```python
from build123d import *

# Parameters (mm, degrees)
SKETCH1_R           = 9
BOSS_EXTRUDE1_DEPTH = 2
SKETCH1_4_W         = 2
SKETCH1_4_H         = 20
BOSS_EXTRUDE2_DEPTH = 8
SKETCH1_5_R         = 0.5
CUT_EXTRUDE1_DEPTH  = 1
CUT_EXTRUDE2_DEPTH  = 9
SKETCH4_R           = 0.5
SKETCH4_R_2         = 1.5
CUT_EXTRUDE5_DEPTH  = 1
SKETCH6_R           = 2.5
CUT_EXTRUDE6_DEPTH  = 10
CUT_EXTRUDE8_DEPTH  = 10


with BuildPart() as part:
    # Sketch1 → Boss-Extrude1 (new body)
    with BuildSketch(Plane(origin=(0, 0, 0), x_dir=(1, 0, 0), z_dir=(0, 1, 0))):
        with Locations(Location((0, 0, 0), (0, 0, 270))):
            Circle(SKETCH1_R)
    extrude(amount=BOSS_EXTRUDE1_DEPTH)

    # Sketch1_4 → Boss-Extrude2 (add)
    with BuildSketch(Plane(origin=(0, 0, 0), x_dir=(1, 0, 0), z_dir=(0, 1, 0))):
        with BuildLine():
            ThreePointArc((9, 0), (6.363961031, -6.363961031), (0, -9))
            Line((0, -9), (14.5, -9))
            Line((14.5, -9), (16.5, -9))
            Line((16.5, -9), (7.566878981, 4.872611465))
            ThreePointArc((7.566878981, 4.872611465), (8.634289514, 2.539496916), (9, 0))
        make_face()
        with Locations((15.5, -19)):
            Rectangle(SKETCH1_4_W, SKETCH1_4_H)
    extrude(amount=BOSS_EXTRUDE2_DEPTH)

    # Sketch1_5 → Cut-Extrude1 (cut)
    with BuildSketch(Plane(origin=(0, 0, 0), x_dir=(1, 0, 0), z_dir=(0, 1, 0))):
        with BuildLine():
            ThreePointArc((2, 1.5), (1.767766953, 1.767766953), (1.5, 2))
            Line((1.5, 2), (1.5, 6.5))
            ThreePointArc((1.5, 6.5), (0, 8), (-1.5, 6.5))
            Line((-1.5, 6.5), (-1.5, 2))
            ThreePointArc((-1.5, 2), (-1.767766953, 1.767766953), (-2, 1.5))
            Line((-2, 1.5), (-6.5, 1.5))
            ThreePointArc((-6.5, 1.5), (-8, 0), (-6.5, -1.5))
            Line((-6.5, -1.5), (-2, -1.5))
            ThreePointArc((-2, -1.5), (-1.767766953, -1.767766953), (-1.5, -2))
            Line((-1.5, -2), (-1.5, -6.5))
            ThreePointArc((-1.5, -6.5), (0, -8), (1.5, -6.5))
            Line((1.5, -6.5), (1.5, -2))
            ThreePointArc((1.5, -2), (1.767766953, -1.767766953), (2, -1.5))
            Line((2, -1.5), (6.5, -1.5))
            ThreePointArc((6.5, -1.5), (8, 0), (6.5, 1.5))
            Line((6.5, 1.5), (2, 1.5))
        make_face()
        with Locations(Location((0, -6.5, 0), (0, 0, 270))):
            Circle(SKETCH1_5_R, mode=Mode.SUBTRACT)
        with Locations(Location((6.5, 0, 0), (0, 0, 270))):
            Circle(SKETCH1_5_R, mode=Mode.SUBTRACT)
        with Locations(Location((0, 6.5, 0), (0, 0, 270))):
            Circle(SKETCH1_5_R, mode=Mode.SUBTRACT)
        with Locations(Location((-6.5, 0, 0), (0, 0, 270))):
            Circle(SKETCH1_5_R, mode=Mode.SUBTRACT)
    extrude(amount=CUT_EXTRUDE1_DEPTH, mode=Mode.SUBTRACT)

    # Sketch2 → Cut-Extrude2 (cut)
    with BuildSketch(Plane.XY.offset(9)):
        Polygon((0, 2), (14.5, 8), (0, 8), align=None)
    extrude(amount=-CUT_EXTRUDE2_DEPTH, mode=Mode.SUBTRACT)

    # Sketch4 → Cut-Extrude5 (cut)
    # profile 1 of 3: a face of its own
    with BuildSketch(Plane(origin=(16.5, 0, 0), x_dir=(0, 0, -1), z_dir=(1, 0, 0))):
        with BuildLine():
            Line((-28.5684803, 6.462476548), (-29, 6.5))
            Line((-29, 6.5), (-29, 1.5))
            Line((-29, 1.5), (-28.5684803, 1.537523452))
            ThreePointArc((-28.5684803, 1.537523452), (-27.085737838, 2.392019784), (-26.5, 4))
            ThreePointArc((-26.5, 4), (-27.085737838, 5.607980216), (-28.5684803, 6.462476548))
        make_face()
    # profile 2 of 3: a face of its own
    with BuildSketch(Plane(origin=(16.5, 0, 0), x_dir=(0, 0, -1), z_dir=(1, 0, 0))):
        with BuildLine():
            Line((-17.5, 5.5), (-28.5684803, 6.462476548))
            ThreePointArc((-28.5684803, 6.462476548), (-27.085737838, 5.607980216), (-26.5, 4))
            ThreePointArc((-26.5, 4), (-27.085737838, 2.392019784), (-28.5684803, 1.537523452))
            Line((-28.5684803, 1.537523452), (-17.5, 2.5))
            ThreePointArc((-17.5, 2.5), (-19, 4), (-17.5, 5.5))
        make_face()
        with Locations((-22.5, 4)):
            Circle(SKETCH4_R, mode=Mode.SUBTRACT)
        with Locations((-20, 4)):
            Circle(SKETCH4_R, mode=Mode.SUBTRACT)
    # profile 3 of 3: a face of its own
    with BuildSketch(Plane(origin=(16.5, 0, 0), x_dir=(0, 0, -1), z_dir=(1, 0, 0))):
        with Locations((-17.5, 4)):
            Circle(SKETCH4_R_2)
        with Locations((-17.5, 4)):
            Circle(SKETCH4_R, mode=Mode.SUBTRACT)
    extrude(amount=-CUT_EXTRUDE5_DEPTH, mode=Mode.SUBTRACT)

    # Sketch6 → Cut-Extrude6 (cut)
    with BuildSketch(Plane(origin=(15.5, 0, 0), x_dir=(0, 0, -1), z_dir=(1, 0, 0))):
        with Locations((-29, 4)):
            Circle(SKETCH6_R)
    extrude(amount=-CUT_EXTRUDE6_DEPTH, mode=Mode.SUBTRACT)

    # Sketch8 → Cut-Extrude8 (cut)
    with BuildSketch(Plane(origin=(16.5, 0, 0), x_dir=(0, 0, -1), z_dir=(1, 0, 0))):
        Polygon((-9, 8), (4.872611465, 2), (4.872611465, 8), align=None)
    extrude(amount=-CUT_EXTRUDE8_DEPTH, mode=Mode.SUBTRACT)


solid = part.part
```
CAD build for the part. Positions are in the model's coordinates, mm. A direction names the side the tool comes from. Round coordinates to 2 decimals unless told otherwise and drop trailing zeros. Write each loop counter-clockwise with the first axis right and the second up, starting at its lowest first coordinate (ties: lowest second). Pieces come first, ordered by that corner, then holes. Notation, with made-up numbers: (-36, -5.5) - (-31, -5.5) arc R13 cw to (-31, 6.5) - close; hole circle Ø10 at (-27, 87.25). An arc over 180 degrees is marked (long way). Write item = value, one per line. Start each with the question number.
Q1. Band-saw the part on C-C (x = -4.25). Give the cut face in (y, z), then the cut area to 3 significant figures.
Q2. Band-saw the part on B-B (y = 3). Give the cut face in (x, z), then the cut area to 3 significant figures.
Q3. Band-saw the part on A-A (z = 7.5). Give the cut face in (x, y).
Q4. Band-saw the part on D-D (z = -2.5). Give the cut face in (x, y).
Q5. Probe L1, parallel to X at y = 0.5, z = 10.5; L2, parallel to Y at x = -7.5, z = 4.5; L3, parallel to X at y = 0.5, z = 6.5. List the from-to ranges inside material, lowest first. Write a range as from..to.
Q6. Drop flat-ended pins along their axis: pin 1 (3 mm diameter, centred on y = 1, z = 3.5, fed in from -X); pin 2 (4 mm diameter, centred on y = 1, z = 15.5, fed in from -X); pin 3 (1.5 mm diameter, centred on x = -2.5, z = -3.5, fed in from +Y). Give the stop position or say it passes through.
Q7. Which spindle directions (+Z, -Z, +X, -X, +Y, -Y) get a long thin tool onto all of the face, cutting with end or side? Do faces 4 (the flat face through (14.5, 4, 19)), 5 (the flat face through (4.3, 0.5, -1.5)), 6 (the flat face through (16.5, 4, 20)). Say none if no direction does.
Q8. Mould opens along Z. For faces 1 (the flat face through (6.5, 0, 0)), 2 (the flat face through (9, 3, 9)), 3 (the cylindrical face through (-0.192, 0.493, 6.962)) say: pulls with the +Z half, pulls with the -Z half, needs draft (parallel to the pull), parting line crosses it, or undercut.
Answers below:
q1.outline = (0, -7.93) - (2, -7.93) - (2, 7.93) - (0, 7.93) - (0, 1.5) - (1, 1.5) - (1, -1.5) - (0, -1.5) - close
q1.area = 28.7 mm2
q2.outline = (2.42, 8.67) arc R9 cw to (8.63, -2.56) - (9.06, -2.56) - (16.5, 9) - (16.5, 16.38) - (15.5, 16.38) - (15.5, 26.71) - (14.5, 26.71) - (14.5, 9) - (2.42, 9) - close
q2.area = 86.2 mm2
q3.outline = (-4.97, 0) - (-1.12, 0) - (-1.12, 1) - (1.12, 1) - (1.12, 0) - (15.53, 0) - (15.53, 7.35) - (12.93, 7.35) - (4.97, 4.06) - (4.97, 2) - (-4.97, 2) - close
q4.outline = (-8.65, 0) - (-1.5, 0) - (-1.5, 1) - (1.5, 1) - (1.5, 0) - (9.09, 0) - (9.09, 3.03) - (8.65, 3.03) - (8.65, 2) - (-8.65, 2) - close
q5.L1 = 14.5..16.5
q5.L2 = 0..2
q5.L3 = -6.22..-1.5, -0.5..0.5, 1.5..14.89
q6.pin_1 = -8.77
q6.pin_2 = 14.5
q6.pin_3 = 2
q7.face_4 = +Z, -X, +Y, -Y
q7.face_5 = -Y
q7.face_6 = +Z, -Z, +X, +Y, -Y
q8.face_1 = needs draft
q8.face_2 = pulls with the +Z half
q8.face_3 = undercut
